Check sheet for the drawn part. Datum: minimum x, y, z corner. Units: mm. A direction names the side the tool comes from. Coordinates: 2 decimals unless noted, no trailing zeros. Loops run counter-clockwise (first coordinate to the right, second up) from the corner with the lowest first, then second, coordinate; pieces in that order, holes last.
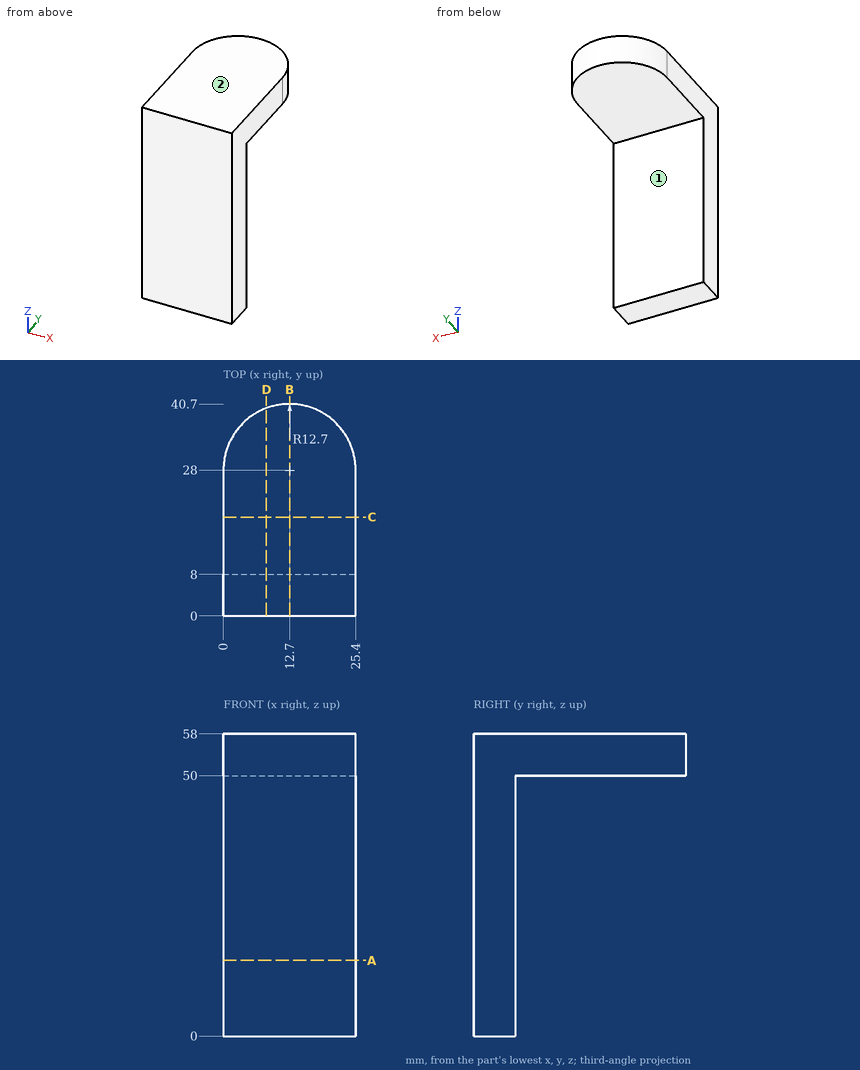
(1) Sectioned sample at C-C on y = 19. Record the cut outline in (x, z).
Findings:
outline: (0, 50) - (25.4, 50) - (25.4, 58) - (0, 58) - close
(2) Sectioned sample at B-B on x = 12.7. Record the cut outline in (y, z).
Findings:
outline: (0, 0) - (8, 0) - (8, 50) - (40.7, 50) - (40.7, 58) - (0, 58) - close
(3) Gauge pin test, flat ends, axial feed: pin 1 Ø4 at (x, z) = (16, 11.5) entering from -Y; pin 2 Ø8 at (y, z) = (12.5, 15.5) entering from +X; pin 3 Ø7.5 at (x, y) = (18, 23.5) entering from -Z; pin 4 Ø12.5 at (x, z) = (8.5, 25.5) entering from +Y. Record the tip position at first contact, or that the pin passes through.
Findings:
pin 1: stops at y = 0
pin 2: passes through
pin 3: stops at z = 50
pin 4: stops at y = 8
(4) Sectioned sample at A-A on z = 14.5. Record the cut outline in (x, y), and give its area (3 significant figures).
Findings:
outline: (0, 0) - (25.4, 0) - (25.4, 8) - (0, 8) - close
area: 203 mm2
(5) Access from +Z, -Z, +X, -X, +Y, -Y to the whole of each face (thin tool, end or side, straight path). Record for the marked faces 1 and 2.
Findings:
face 1: -Z, +X, -X, +Y
face 2: +Z, +X, -X, +Y, -Y
(6) Sectioned sample at D-D on x = 8.25. Record the cut outline in (y, z).
Findings:
outline: (0, 0) - (8, 0) - (8, 50) - (39.89, 50) - (39.89, 58) - (0, 58) - close
(7) Scan lines: L1, parallel to Y at x = 22, z = 36; L2, parallel to Z at x = 16.25, y = 37.5; L3, parallel to Y at x = 11.5, z = 52. Record each from-to range of solid material in increasing order.
Findings:
L1: y = 0 to 8
L2: z = 50 to 58
L3: y = 0 to 40.64
